Build history of the part. All positions in model axes, mm. Give positions to 0.01 mm unless a question says otherwise; leave off trailing zeros. Order: outer loops, then holes, each group sorted by start corner. A loop starts at its lowest first (then second) coordinate and runs counter-clockwise, first axis right, second up. Notation, with made-up numbers: (-10.5, -37.75) - (38.5, -37.75) arc R35 ccw to (38.5, -0.75) - close; hole circle Ø11 at (-18, 76). An arc over 180 degrees is marked (long way). Use a Markdown table: item, result.
from build123d import *

# Parameters (mm, degrees)
SKETCH1_W           = 88.9
SKETCH1_H           = 147
BOSS_EXTRUDE1_DEPTH = 25.4
SKETCH2_R           = 1.74244
CUT_EXTRUDE1_DEPTH  = 30
CUT_EXTRUDE2_REACH  = 90.9
SKETCH3_R           = 2


with BuildPart() as part:
    # Sketch1 → Boss-Extrude1 (new body)
    with BuildSketch(Plane(origin=(0, 0, 0), x_dir=(1, 0, 0), z_dir=(0, 1, 0))):
        Rectangle(SKETCH1_W, SKETCH1_H)
    extrude(amount=BOSS_EXTRUDE1_DEPTH)

    # Sketch2 → Cut-Extrude1 (cut)
    with BuildSketch(Plane.XZ):
        with Locations((41.27, -32.22)):
            Circle(SKETCH2_R)
        with Locations((41.27, 12.23)):
            Circle(SKETCH2_R)
        with Locations((-41.27, -32.22)):
            Circle(SKETCH2_R)
        with Locations((-41.27, 12.23)):
            Circle(SKETCH2_R)
    extrude(amount=-CUT_EXTRUDE1_DEPTH, mode=Mode.SUBTRACT)

    # Sketch3 → Cut-Extrude2 (cut, up to next)
    with BuildSketch(Plane(origin=(44.45, 0, 0), x_dir=(0, 0, -1), z_dir=(1, 0, 0)), mode=Mode.PRIVATE) as cut_extrude2_sk1:
        with Locations((-59.1, 4.5)):
            Circle(SKETCH3_R)
    cut_extrude2_tool1 = extrude(cut_extrude2_sk1.sketch, amount=-CUT_EXTRUDE2_REACH, mode=Mode.PRIVATE) & part.part
    add(cut_extrude2_tool1.solids().sort_by_distance((44.45, 4.5, 59.1))[0], mode=Mode.SUBTRACT)
    # Sketch3 → Cut-Extrude2 (cut, up to next)
    with BuildSketch(Plane(origin=(44.45, 0, 0), x_dir=(0, 0, -1), z_dir=(1, 0, 0)), mode=Mode.PRIVATE) as cut_extrude2_sk2:
        with Locations((43.2, 4.5)):
            Circle(SKETCH3_R)
    cut_extrude2_tool2 = extrude(cut_extrude2_sk2.sketch, amount=-CUT_EXTRUDE2_REACH, mode=Mode.PRIVATE) & part.part
    add(cut_extrude2_tool2.solids().sort_by_distance((44.45, 4.5, -43.2))[0], mode=Mode.SUBTRACT)


solid = part.part
1) Wall check: line 1 (Y direction, x = 8, z = -43); line 2 (Y direction, x = -11, z = 58). Give the ranges that are in metal, low to high. Write a range as from..to.
Computed:
| item | result |
|---|---|
| line 1 | y = 0..2.51, 6.49..25.4 |
| line 2 | y = 0..2.83, 6.17..25.4 |
2) Slice it at C-C (z = -32.22). Write the cut outline in (x, y).
Computed:
| item | result |
|---|---|
| outline | (-44.45, 0) - (-43.01, 0) - (-43.01, 25.4) - (-44.45, 25.4) - close; (-39.53, 0) - (39.53, 0) - (39.53, 25.4) - (-39.53, 25.4) - close; (43.01, 0) - (44.45, 0) - (44.45, 25.4) - (43.01, 25.4) - close |
3) Slice it at A-A (x = 41.27). Write the cut outline in (y, z).
Computed:
| item | result |
|---|---|
| outline | (0, -73.5) - (25.4, -73.5) - (25.4, -33.96) - (0, -33.96) - close; (0, -30.48) - (25.4, -30.48) - (25.4, 10.49) - (0, 10.49) - close; (0, 13.97) - (25.4, 13.97) - (25.4, 73.5) - (0, 73.5) - close; hole circle Ø4 at (4.5, -43.2); hole circle Ø4 at (4.5, 59.1) |
4) Two-plate mould, pull along X, no slides. Class faces 1 (the flat face through (-1, 13, 73.5)), 2 (the cylindrical face through (-42.653, 12.522, 11.17)), 3 (the flat face through (-44.45, 13, 1)): +X half, -X half, draft (parallel to the pull), parting line (faces both ways), or undercut.
Computed:
| item | result |
|---|---|
| face 1 | draft |
| face 2 | undercut |
| face 3 | -X half |
5) Slice it at B-B (z = 59.1). Write the cut outline in (x, y).
Computed:
| item | result |
|---|---|
| outline | (-44.45, 0) - (44.45, 0) - (44.45, 2.5) - (-44.45, 2.5) - close; (-44.45, 6.5) - (44.45, 6.5) - (44.45, 25.4) - (-44.45, 25.4) - close |
6) Pin check, flat tips, straight feed: P1, Ø2, axis at x = 41.27, z = 12.23, coming from the +Y side; P2, Ø5, axis at y = 4.5, z = -43.2, coming from the -X side. Stop position of each tip, or through.
Computed:
| item | result |
|---|---|
| P1 | passes through |
| P2 | stops at x = -44.45 |
